Can you work these out from the model? Positions are in its coordinate system, mm. Round coordinates to 2 decimals unless told otherwise and drop trailing zeros. Write each loop counter-clockwise with the first axis right and the second up, starting at its lowest first coordinate (ties: lowest second). Pieces come first, ordered by that corner, then holes. Notation, with made-up numbers: M 60,67 L 73,67 A20 ccw 73,82 Z; hole C 41.25,12.5 d8. An arc over 180 degrees is marked long. Answer as a JSON object with one key per item and string values. Group by question number.
1) Please list where these lines run through material, in increasing order: L1, parallel to Z at x = 1.2, y = -1; L2, parallel to Z at x = 1.1, y = 6; L3, parallel to Z at x = 1, y = 11. Write a range as [from, to].
2) Suppose I cut it at B-B, the plane y = 17.5. Write out the boundary of the cut face in (x, z), and give its area (3 significant figures).
3) Suppose I cut it at A-A, the plane x = 0.7. Write out the boundary of the cut face in (y, z) (3 decimals), and give its area (3 significant figures).
4) If we mould it in two halves opening along Y, with no side actions, what happens to faces 1 (the flat face through (0.78, 19.55, -108.07)), 2 (the cylindrical face through (0.78, -26.92, 101.55)), 3 (the cylindrical face through (0.78, -26.47, -100.23)), 4 (the flat face through (0, 0, 2))? For each: +Y half, -Y half, draft (parallel to the pull), parting line (faces both ways), or undercut.
5) I'm going to push a flat-ended pin straight in: pin 1 Ø2.5 at (y, z) = (0.66, -101.56) entering from -X. Where does the tip first touch, or does it pass through?
6) Suppose I cut it at C-C, the plane y = 28. Write out the boundary of the cut face in (x, z).
Autodesk Inventor part; units mm, degrees
ref_plane "YZ Plane" through (0, 0, 0) normal (1, 0, 0) x (0, 1, 0)
ref_plane "XZ Plane" through (0, 0, 0) normal (0, 1, 0) x (-1, 0, 0)
ref_plane "XY Plane" through (0, 0, 0) normal (0, 0, 1) x (1, 0, 0)
sketch "Sketch1" plane through (0, 0, 0) normal (1, 0, 0) x (0, 1, 0)
  line L0 (-31.0872, -5.216) -> (-31.0872, 56.252)
  line L1 (-31.0872, -117.4332) -> (-31.0872, 117.5168)
  line L2 (-27.9122, 120.6918) -> (5.6976, 120.6918)
  line L3 (-27.9122, -120.6082) -> (5.6976, -120.6082)
  line L4 (32.4128, 93.9766) -> (32.4128, -93.8931)
  line L5 (7.9427, 119.7618) -> (31.4828, 96.2217)
  line L6 (7.9427, -119.6783) -> (31.4828, -96.1382)
  arc A0 (32.4128, 93.9766) -> (31.4828, 96.2217) centre (29.2378, 93.9766) ccw
  arc A1 (31.4828, -96.1382) -> (32.4128, -93.8931) centre (29.2378, -93.8931) ccw
  arc A2 (5.6976, -120.6082) -> (7.9427, -119.6783) centre (5.6976, -117.4332) ccw
  arc A3 (-31.0872, -117.4332) -> (-27.9122, -120.6082) centre (-27.9122, -117.4332) ccw
  arc A4 (-27.9122, 120.6918) -> (-31.0872, 117.5168) centre (-27.9122, 117.5168) ccw
  arc A5 (7.9427, 119.7618) -> (5.6976, 120.6918) centre (5.6976, 117.5168) ccw
  circle A6 centre (0.6628, 101.6418) radius 2.1844
  circle A7 centre (-24.7372, 101.6418) radius 2.1844
  circle A8 centre (-24.7372, -101.5582) radius 2.1844
  circle A9 centre (0.6628, -101.5582) radius 2.1844
  point P0 (0, 0)
  point P1 (-31.0872, -120.6082)
  point P2 (-31.0872, 120.6918)
  point P3 (7.0128, 120.6918)
  point P4 (7.0128, -120.6082)
  dimension "d0" = 241.3
  dimension "d1" = 38.1
  dimension "d2" = 38.1
  dimension "d3" = 3.175
  dimension "d4" = 3.175
  dimension "d5" = 3.175
  dimension "d6" = 3.175
  dimension "d7" = 3.175
  dimension "d8" = 3.175
  dimension "d15" = 4.3688
  dimension "d16" = 4.3688
  dimension "d17" = 4.3688
  dimension "d18" = 4.3688
extrude "Extrusion1" add sketch "Sketch1" along normal blind 1.5875
properties part number "wedge"
Results:
{
 "1": {"L1": "[-120.61, -102.97], [-100.14, 100.23], [103.06, 120.69]", "L2": "[-120.59, 120.68]", "L3": "[-116.62, 116.7]"},
 "2": {"outline": "M 0,-110.12 L 1.59,-110.12 L 1.59,110.2 L 0,110.2 Z", "area": "350 mm^2"},
 "3": {"outline": "M -31.087,-117.433 A3.175 ccw -27.912,-120.608 L 5.698,-120.608 A3.175 ccw 7.943,-119.678 L 31.483,-96.138 A3.175 ccw 32.413,-93.893 L 32.413,93.977 A3.175 ccw 31.483,96.222 L 7.943,119.762 A3.175 ccw 5.698,120.692 L -27.912,120.692 A3.175 ccw -31.087,117.517 Z; hole C -24.737,-101.558 d4.369; hole C -24.737,101.642 d4.369; hole C 0.663,-101.558 d4.369; hole C 0.663,101.642 d4.369", "area": "14,600 mm^2"},
 "4": {"face 1": "+Y half", "face 2": "undercut", "face 3": "undercut", "face 4": "draft"},
 "5": {"pin 1": "through"},
 "6": {"outline": "M 0,-99.62 L 1.59,-99.62 L 1.59,99.7 L 0,99.7 Z"}
}
